Source: CAD feature listing. Evaluate the final solid. Frame: model axes, mm. Face numbers are marked on the shaded views. A direction names the side the tool comes from. Give positions to 0.01 mm unless a question says otherwise; leave off trailing zeros. Order: outer loops, then holes, each group sorted by start corner. A loop starts at its lowest first (then second) coordinate and runs counter-clockwise, first axis right, second up. Notation, with made-up numbers: M 30,3 L 50,3 A8 ccw 50,11 Z; hole C 87.25,61 d1. An arc over 180 degrees is marked long. Answer as a JSON object with one key per item and string values. Group by question number.
1. Section query A-A (z = 16.25). Output: boundary loops of the cut face in (x, y) (3 decimals), plus the area to 3 significant figures.
2. Section query C-C (y = 2.3). Output: boundary loops of the cut face in (x, z) (3 decimals).
3. Section query D-D (x = 5.5). Output: boundary loops of the cut face in (y, z), plus the area to 3 significant figures.
4. Set-up query: the marked faces 1, 2, 3 and 4. Return all of +Z, -Z, +X, -X, +Y, -Y with unobstructed straight access to the full face (end or side cutting, diameter ignored); none if empty.
5. Pin query (flat end, axial travel): P1, Ø4, axis at x = -30, z = 11.5, coming from the -Y side; P2, Ø4.5, axis at y = 35.5, z = 14, coming from the +X side (3 decimals); P3, Ø10.5, axis at x = 27, z = 17, coming from the -Y side. Return the tip coordinate at first contact, or that it passes through.
6. Section query B-B (z = 5). Output: boundary loops of the cut face in (x, y) (3 decimals), plus the area to 3 significant figures.
7. Material intervals for L1, parallel to X at y = 44.5, z = 15.25 (3 decimals); L2, parallel to Z at x = -8, y = -28.5; L3, parallel to Z at x = 10, y = 46, sorted ascending. Write a range as [from, to].
from build123d import *

# Parameters (mm, degrees)
SKETCH1_W           = 85.09
SKETCH1_H           = 85.6
SKETCH1_R           = 2
BOSS_EXTRUDE1_DEPTH = 8
SKETCH2_W           = 13
SKETCH2_H           = 17
SKETCH2_W_2         = 14
SKETCH2_H_2         = 9
BOSS_EXTRUDE2_DEPTH = 14.25
SKETCH3_R           = 2.5
CUT_EXTRUDE1_DEPTH  = 3
SKETCH4_W           = 28.5
SKETCH4_H           = 10
BOSS_EXTRUDE3_DEPTH = 85


with BuildPart() as part:
    # Sketch1 → Boss-Extrude1 (new body)
    with BuildSketch(Plane.XY):
        Rectangle(SKETCH1_W, SKETCH1_H)
        with Locations((-32.045, 32.8)):
            Circle(SKETCH1_R, mode=Mode.SUBTRACT)
        with Locations((38.545, 32.8)):
            Circle(SKETCH1_R, mode=Mode.SUBTRACT)
        with Locations((38.545, -35.8)):
            Circle(SKETCH1_R, mode=Mode.SUBTRACT)
        with Locations((-32.045, -35.8)):
            Circle(SKETCH1_R, mode=Mode.SUBTRACT)
    extrude(amount=BOSS_EXTRUDE1_DEPTH)

    # Sketch2 → Boss-Extrude2 (add)
    with BuildSketch(Plane.XY.offset(8)):
        with Locations((26.745, 39.3)):
            Rectangle(SKETCH2_W, SKETCH2_H)
        with Locations((4.245, 39.3)):
            Rectangle(SKETCH2_W, SKETCH2_H)
        with Locations((-18.255, 39.3)):
            Rectangle(SKETCH2_W, SKETCH2_H)
        with Locations((-35.545, 2.3)):
            Rectangle(SKETCH2_W_2, SKETCH2_H_2)
    extrude(amount=BOSS_EXTRUDE2_DEPTH)

    # Sketch3 → Cut-Extrude1 (cut)
    with BuildSketch(Plane.ZY.offset(42.545)):
        with Locations((16.25, 2.3)):
            Circle(SKETCH3_R)
    extrude(amount=-CUT_EXTRUDE1_DEPTH, mode=Mode.SUBTRACT)

    # Sketch4 → Boss-Extrude3 (add)
    with BuildSketch(Plane(origin=(0, 47.8, 0), x_dir=(1, 0, 0), z_dir=(0, 1, 0))):
        with Locations((26.745, -17.25)):
            Rectangle(SKETCH4_W, SKETCH4_H)
    extrude(amount=BOSS_EXTRUDE3_DEPTH)


solid = part.part
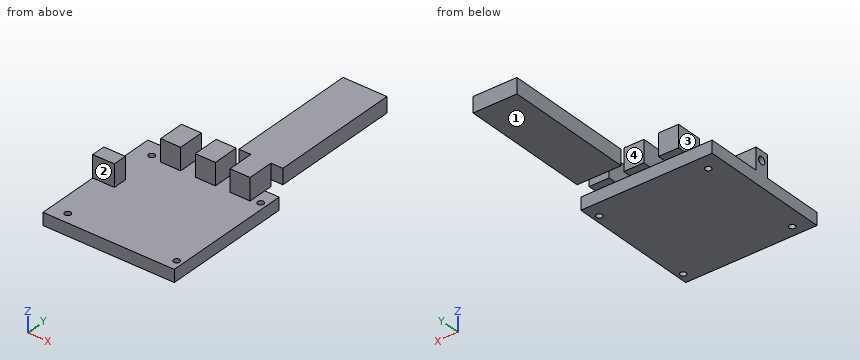
Answer sheet:
{
 "1": {"outline": "M -42.545,-2.2 L -28.545,-2.2 L -28.545,6.8 L -42.545,6.8 L -42.545,4.8 L -39.545,4.8 L -39.545,-0.2 L -42.545,-0.2 Z; M -24.755,30.8 L -11.755,30.8 L -11.755,47.8 L -24.755,47.8 Z; M -2.255,30.8 L 10.745,30.8 L 10.745,47.8 L -2.255,47.8 Z; M 12.495,47.8 L 20.245,47.8 L 20.245,30.8 L 33.245,30.8 L 33.245,47.8 L 40.995,47.8 L 40.995,132.8 L 12.495,132.8 Z", "area": "3,200 mm^2"},
 "2": {"outline": "M -42.545,0 L 42.545,0 L 42.545,8 L -28.545,8 L -28.545,22.25 L -42.545,22.25 L -42.545,18.75 L -39.545,18.75 L -39.545,13.75 L -42.545,13.75 Z"},
 "3": {"outline": "M -42.8,0 L 42.8,0 L 42.8,8 L 47.8,8 L 47.8,22.25 L 30.8,22.25 L 30.8,8 L -42.8,8 Z", "area": "927 mm^2"},
 "4": {"face 1": "-Z, +X, -X, +Y", "face 2": "+Z, +X, -X, -Y", "face 3": "+Z, -X, +Y, -Y", "face 4": "+Z, -Z, -X, +Y"},
 "5": {"P1": "y = -2.2", "P2": "x = 33.245", "P3": "y = 30.8"},
 "6": {"outline": "M -42.545,-42.8 L 42.545,-42.8 L 42.545,42.8 L -42.545,42.8 Z; hole C -32.045,-35.8 d4; hole C -32.045,32.8 d4; hole C 38.545,-35.8 d4; hole C 38.545,32.8 d4", "area": "7,230 mm^2"},
 "7": {"L1": "[-24.755, -11.755], [-2.255, 10.745], [20.245, 33.245]", "L2": "[0, 8]", "L3": "[8, 22.25]"}
}
